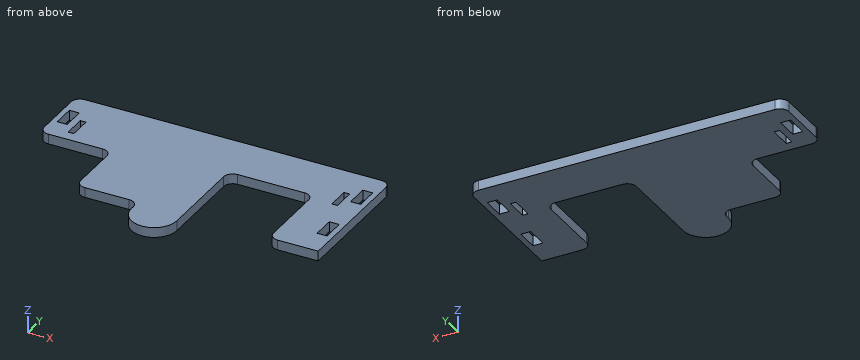
```python
from build123d import *

# Parameters (mm, degrees)
BOSS_EXTRUDE1_DEPTH = 2.794
SKETCH3_W           = 2.794
SKETCH3_H           = 6.35
SKETCH3_W_2         = 1.5875
CUT_EXTRUDE1_DEPTH  = 78.110446656
FILLET1_R           = 2.54


with BuildPart() as part:
    # Sketch1 → Boss-Extrude1 (new body)
    with BuildSketch(Plane.XY):
        with BuildLine():
            Line((69.475359958, -4.3815), (69.475359958, 33.3375))
            Line((69.475359958, 33.3375), (-18.662640042, 33.3375))
            Line((-18.662640042, 33.3375), (-18.662640042, 14.2875))
            Line((-18.662640042, 14.2875), (1.5875, 14.2875))
            Line((1.5875, 14.2875), (1.5875, -4.3815))
            Line((1.5875, -4.3815), (19.056359958, -4.3815))
            Line((19.056359958, -4.3815), (19.056359958, -7.8778))
            ThreePointArc((19.056359958, -7.8778), (25.406359958, -14.2278), (31.756359958, -7.8778))
            Line((31.756359958, -7.8778), (31.756359958, 19.05))
            Line((31.756359958, 19.05), (55.568859958, 19.05))
            Line((55.568859958, 19.05), (55.568859958, -4.3815))
            Line((55.568859958, -4.3815), (69.475359958, -4.3815))
        make_face()
    extrude(amount=BOSS_EXTRUDE1_DEPTH)

    # Sketch3 → Cut-Extrude1 (cut, through all)
    with BuildSketch(Plane.XY.offset(2.794)):
        with Locations((-15.678140042, 23.8125)):
            Rectangle(SKETCH3_W, SKETCH3_H)
        with Locations((66.490859958, 23.8125)):
            Rectangle(SKETCH3_W, SKETCH3_H)
        with Locations((66.490859958, 6.35)):
            Rectangle(SKETCH3_W, SKETCH3_H)
        with Locations((-11.518890042, 20.6375)):
            Rectangle(SKETCH3_W_2, SKETCH3_H)
        with Locations((62.331609958, 20.6375)):
            Rectangle(SKETCH3_W_2, SKETCH3_H)
    extrude(amount=-CUT_EXTRUDE1_DEPTH, mode=Mode.SUBTRACT)

    # Fillet1
    fillet1_edges = [part.edges().sort_by_distance(p)[0] for p in [
        (55.568859958, -4.3815, 1.397),
        (55.568859958, 19.05, 1.397),
        (31.756359958, 19.05, 1.397),
        (19.056359958, -4.3815, 1.397),
        (1.5875, -4.3815, 1.397),
        (1.5875, 14.2875, 1.397),
        (-18.662640042, 14.2875, 1.397),
        (-18.662640042, 33.3375, 1.397),
        (69.475359958, 33.3375, 1.397),
    ]]
    fillet(fillet1_edges, radius=FILLET1_R)


solid = part.part
```
Could you check a few things on this model? Use its own coordinates, in mm. Round coordinates to 2 decimals unless told otherwise and drop trailing zeros. Loops run counter-clockwise (first coordinate to the right, second up) from the corner with the lowest first, then second, coordinate; pieces in that order, holes last. Notation, with made-up numbers: (11.5, 82) - (60.5, 82) arc R16 cw to (60.5, 106) - close; hole circle Ø3 at (-14, 12). An arc over 180 degrees is marked (long way). Answer as CSV lines item,"result".
1. I want a section at D-D on z = 1.7. Count the separate pieces of the cut face and the enclosed holes in it, then the cut area to 3 significant figures.
Filled in:
separate pieces,"1"
enclosed holes,"5"
area,"2,420 mm^2"
2. Please list where these lines run through material, in increasing order: line 1 along X through (y, z) = (8, 1.9); line 2 along X through (y, z) = (23, 0.55); line 3 along X through (y, z) = (0, 2.5). Write a range as [from, to].
Filled in:
line 1,"x = [1.59, 31.76], [55.57, 65.09], [67.89, 69.48]"
line 2,"x = [-18.66, -17.08], [-14.28, -12.31], [-10.73, 61.54], [63.13, 65.09], [67.89, 69.48]"
line 3,"x = [1.59, 31.76], [55.57, 69.48]"
3. I want a section at A-A on y = 2. List the corners of the cut face in (x, z) for me.
Filled in:
outline,"(1.59, 0) - (31.76, 0) - (31.76, 2.79) - (1.59, 2.79) - close; (55.57, 0) - (69.48, 0) - (69.48, 2.79) - (55.57, 2.79) - close"
4. I want a section at C-C on x = 43. List the corners of the cut face in (y, z) for me, then the cut area to 3 significant figures.
Filled in:
outline,"(19.05, 0) - (33.34, 0) - (33.34, 2.79) - (19.05, 2.79) - close"
area,"39.9 mm^2"
5. For pin 1 Ø1 at (y, z) = (7.5, 0.5) entering from -X; pin 2 Ø1.1 at (y, z) = (-7.5, 2) entering from -X; pin 3 Ø5 at (x, y) = (10.5, -7.5) entering from -Z; pin 4 Ø0.8 at (x, z) = (-9, 1) entering from -Y, each with a flat end and sliding along its axis, tell me the tip position at first contact or that it passes through.
Filled in:
pin 1,"stops at x = 1.59"
pin 2,"stops at x = 19.06"
pin 3,"passes through"
pin 4,"stops at y = 14.29"
6. I want a section at B-B on y = 8. List the corners of the cut face in (x, z) for me, then the cut area to 3 significant figures.
Filled in:
outline,"(1.59, 0) - (31.76, 0) - (31.76, 2.79) - (1.59, 2.79) - close; (55.57, 0) - (65.09, 0) - (65.09, 2.79) - (55.57, 2.79) - close; (67.89, 0) - (69.48, 0) - (69.48, 2.79) - (67.89, 2.79) - close"
area,"115 mm^2"
